Design review of the part shown in the three views and the two pictorial views. Dimensions are in mm from the part's minimum x, y and z. A direction names the side the tool comes from. Coordinates: 2 decimals unless noted, no trailing zeros. Order: outer loops, then holes, each group sorted by start corner. A loop starts at its lowest first (then second) coordinate and runs counter-clockwise, first axis right, second up. Notation, with made-up numbers: (20, 76.5) -> (58, 76.5) arc R34 cw to (58, 114.5) -> close; hole circle Ø9 at (-33.75, -10). An arc over 180 degrees is marked (long way). Answer as a JSON object with one key per item and string values. Group by question number.
1) Draft analysis for pull direction X (two halves, no side actions). For the marked faces 1, 2, 3 and 4, state which applies: +X half, -X half, draft (parallel to the pull), parting line (faces both ways), or undercut.
2) Add section A-A, the plane y = 8. Write out the cut boundary in (x, z).
3) Wall thickness on L1, parallel to X at y = 11.25, z = 3.25; L2, parallel to Y at x = 14, z = 11; L3, parallel to X at y = 1.4, z = 10: over which ranges is each line inside the solid? List them lowest first.
4) Machinability: for the marked faces 5 and 6, which of the approach directions +Z, -Z, +X, -X, +Y, -Y give a long, thin tool a straight path to every point of the face, cutting with its end or side? Answer none if there is none.
5) Add section D-D, the plane z = 5. Write out the cut boundary in (x, y).
6) Add section C-C, the plane z = 10. Write out the cut boundary in (x, y).
7) For pin 1 (9 mm diameter, centred on x = 21.5, z = 10, fed in from -Y); pin 2 (6 mm diameter, centred on x = 24, z = 15, fed in from +Y); pin 3 (2 mm diameter, centred on y = 4.5, z = 4.5, fed in from -X), all flat-tipped, find the tip position at first contact; note any pin that passes through.
8) Add section B-B, the plane x = 21.5. Write out the cut boundary in (y, z).
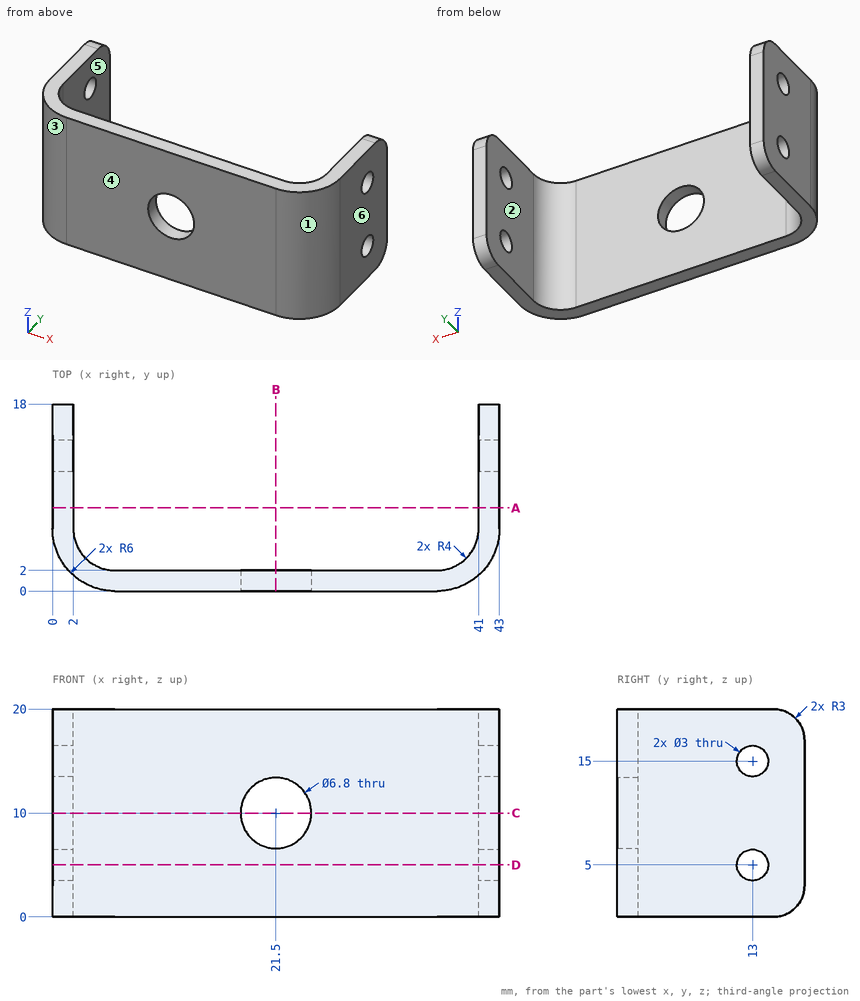
Output values:
{
 "1": {"face 1": "+X half", "face 2": "undercut", "face 3": "-X half", "face 4": "draft"},
 "2": {"outline": "(0, 0) -> (2, 0) -> (2, 20) -> (0, 20) -> close; (41, 0) -> (43, 0) -> (43, 20) -> (41, 20) -> close"},
 "3": {"L1": "x = 0 to 2, 41 to 43", "L2": "y = 0 to 2", "L3": "x = 2.15 to 18.1, 24.9 to 40.85"},
 "4": {"face 5": "+Z, -Z, +Y", "face 6": "+Z, -Z, +X, +Y, -Y"},
 "5": {"outline": "(0, 6) arc R6 ccw to (6, 0) -> (37, 0) arc R6 ccw to (43, 6) -> (43, 11.5) -> (41, 11.5) -> (41, 6) arc R4 cw to (37, 2) -> (6, 2) arc R4 cw to (2, 6) -> (2, 11.5) -> (0, 11.5) -> close; (0, 14.5) -> (2, 14.5) -> (2, 18) -> (0, 18) -> close; (41, 14.5) -> (43, 14.5) -> (43, 18) -> (41, 18) -> close"},
 "6": {"outline": "(0, 6) arc R6 ccw to (6, 0) -> (18.1, 0) -> (18.1, 2) -> (6, 2) arc R4 cw to (2, 6) -> (2, 18) -> (0, 18) -> close; (24.9, 0) -> (37, 0) arc R6 ccw to (43, 6) -> (43, 18) -> (41, 18) -> (41, 6) arc R4 cw to (37, 2) -> (24.9, 2) -> close"},
 "7": {"pin 1": "stops at y = 0", "pin 2": "stops at y = 2", "pin 3": "stops at x = 0.02"},
 "8": {"outline": "(0, 0) -> (2, 0) -> (2, 6.6) -> (0, 6.6) -> close; (0, 13.4) -> (2, 13.4) -> (2, 20) -> (0, 20) -> close"}
}
